Design review of the part built by this model. Coordinates are the model's own, in mm. Face numbers are marked on the shaded views. Coordinates: 2 decimals unless noted, no trailing zeros. Write each loop counter-clockwise with the first axis right and the second up, starting at its lowest first coordinate (ties: lowest second). Pieces come first, ordered by that corner, then holes. Notation, with made-up numbers: (39.5, -14.75) - (81.5, -14.75) arc R15 ccw to (81.5, -5.75) - close; hole circle Ø4 at (-31, 29.25). An arc over 180 degrees is marked (long way). Answer as a JSON object with one key per item and string values.
Autodesk Inventor part; units mm, degrees
ref_plane "YZ Plane" through (0, 0, 0) normal (1, 0, 0) x (0, 1, 0)
ref_plane "XZ Plane" through (0, 0, 0) normal (0, 1, 0) x (-1, 0, 0)
ref_plane "XY Plane" through (0, 0, 0) normal (0, 0, 1) x (1, 0, 0)
sketch "Sketch1" plane through (0, 0, 0) normal (0, 0, 1) x (1, 0, 0)
  circle A0 centre (23.8125, 0) radius 2.1463
  circle A1 centre (11.9063, 20.6222) radius 2.1463
  circle A2 centre (-11.9062, 20.6222) radius 2.1463
  circle A3 centre (-23.8125, 0) radius 2.1463
  circle A4 centre (-11.9063, -20.6222) radius 2.1463
  circle A5 centre (11.9062, -20.6222) radius 2.1463
  circle A6 centre (0, 0) radius 38.1
  circle A7 centre (0, 0) radius 7.62
  dimension "d0" = 4.2926
  dimension "d4" = 360
  dimension "d6" = 76.2
  dimension "d9" = 15.24
extrude "Extrusion1" add sketch "Sketch1" along normal mid plane 12.7
properties part number "Spool Hub" material "Acetal Resin, White"
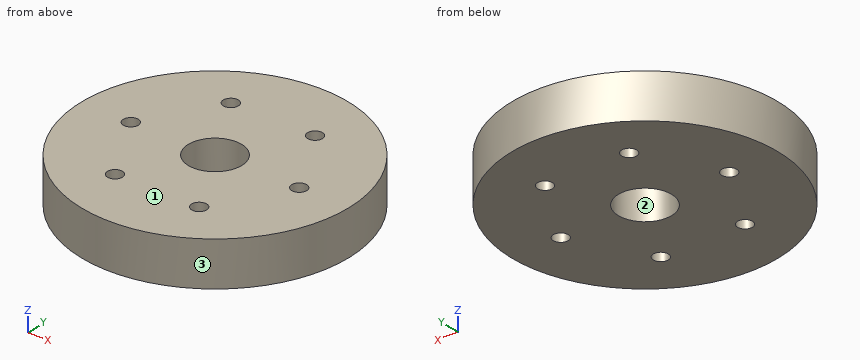
(1) For pin 1 (1 mm diameter, centred on y = -3, z = -4.5, fed in from -X); pin 2 (1.5 mm diameter, centred on y = -23, z = -2.5, fed in from +X); pin 3 (1.5 mm diameter, centred on x = -19.5, z = 1.5, fed in from +Y); pin 4 (3.5 mm diameter, centred on x = 23.81, y = 0, fed in from -Z), all flat-tipped, find the tip position at first contact; note any pin that passes through.
Solved:
{"pin 1": "stops at x = -38.02", "pin 2": "stops at x = 30.93", "pin 3": "stops at y = 33.17", "pin 4": "passes through"}
(2) To check wall thickness, follow line 1 (Y direction, x = 0, z = 0.25); line 2 (X direction, y = -20, z = -5.5); line 3 (X direction, y = 1.5, z = -3). State the ranges of each line that lie inside material, in increasing order. Write a range as from..to.
Solved:
{"line 1": "y = -38.1..-7.62, 7.62..38.1", "line 2": "x = -32.43..-13.96, -9.85..9.85, 13.96..32.43", "line 3": "x = -38.07..-25.35, -22.28..-7.47, 7.47..22.28, 25.35..38.07"}
(3) Take a section at C-C, the plane x = -11. Write out the cut boundary in (y, z).
Solved:
{"outline": "(-36.48, -6.35) - (-22.57, -6.35) - (-22.57, 6.35) - (-36.48, 6.35) - close; (-18.68, -6.35) - (18.68, -6.35) - (18.68, 6.35) - (-18.68, 6.35) - close; (22.57, -6.35) - (36.48, -6.35) - (36.48, 6.35) - (22.57, 6.35) - close"}
(4) Take a section at D-D, the plane z = -4.5. Write out the cut boundary in (x, y), and give its area (3 significant figures).
Solved:
{"outline": "circle Ø76.2 at (0, 0); hole circle Ø4.29 at (-23.81, 0); hole circle Ø4.29 at (-11.91, -20.62); hole circle Ø4.29 at (-11.91, 20.62); hole circle Ø15.24 at (0, 0); hole circle Ø4.29 at (11.91, -20.62); hole circle Ø4.29 at (11.91, 20.62); hole circle Ø4.29 at (23.81, 0)", "area": "4,290 mm^2"}
(5) Take a section at A-A, the plane x = 0. Write out the cut boundary in (y, z).
Solved:
{"outline": "(-38.1, -6.35) - (-7.62, -6.35) - (-7.62, 6.35) - (-38.1, 6.35) - close; (7.62, -6.35) - (38.1, -6.35) - (38.1, 6.35) - (7.62, 6.35) - close"}
(6) Take a section at B-B, the plane y = 0. Write out the cut boundary in (x, z).
Solved:
{"outline": "(-38.1, -6.35) - (-25.96, -6.35) - (-25.96, 6.35) - (-38.1, 6.35) - close; (-21.67, -6.35) - (-7.62, -6.35) - (-7.62, 6.35) - (-21.67, 6.35) - close; (7.62, -6.35) - (21.67, -6.35) - (21.67, 6.35) - (7.62, 6.35) - close; (25.96, -6.35) - (38.1, -6.35) - (38.1, 6.35) - (25.96, 6.35) - close"}
(7) The part is to be moulded in two halves that separate along Y. For the marked faces 1, 2 and 3, say which applies: pulls with the +Y half, pulls with the -Y half, needs draft (parallel to the pull), parting line crosses it, or undercut.
Solved:
{"face 1": "needs draft", "face 2": "undercut", "face 3": "parting line crosses it"}
